Verification items for this drawing (mm, ordinates from the low corner). A direction names the side the tool comes from. Coordinates: 2 decimals unless noted, no trailing zeros. Order: outer loops, then holes, each group sorted by start corner. A loop starts at its lowest first (then second) coordinate and runs counter-clockwise, first axis right, second up. Notation, with made-up numbers: (50, -32.5) -> (91, -32.5) arc R32 ccw to (91, -6.5) -> close; hole circle Ø8 at (49, 88). An arc over 180 degrees is marked (long way). Put each result on its own line as item: value. Start each with the question number.
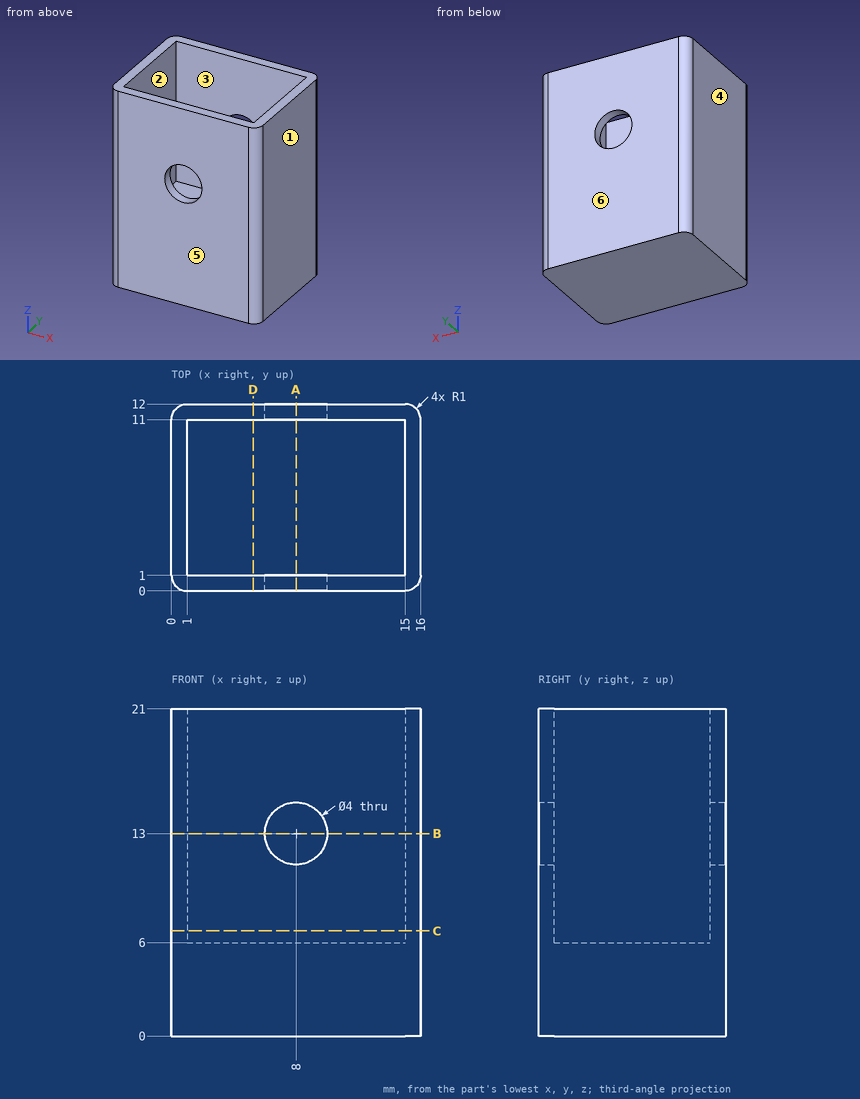
1) Mould release check, pull along Y, two halves, no side actions. Record for the marked faces 3, 4, 5 and 6: +Y half, -Y half, draft (parallel to the pull), parting line (faces both ways), or undercut.
2) Gauge pin test, flat ends, axial feed: pin 1 (4 mm diameter, centred on x = 4, y = 5.5, fed in from +Z); pin 2 (6.5 mm diameter, centred on x = 8, z = 13, fed in from -Y); pin 3 (3.5 mm diameter, centred on x = 8, z = 13, fed in from -Y) (3 decimals). Record the tip position at first contact, or that the pin passes through.
3) Sectioned sample at D-D (x = 5.25). Record the boundary of the cut face in (y, z), plus the area to 3 significant figures.
4) Access from +Z, -Z, +X, -X, +Y, -Y to the whole of each face (thin tool, end or side, straight path). Record for the marked faces 1 and 2.
5) Sectioned sample at A-A (x = 8). Record the boundary of the cut face in (y, z).
6) Sectioned sample at B-B (z = 13). Record the boundary of the cut face in (x, y).
7) Sectioned sample at C-C (z = 6.75). Record the boundary of the cut face in (x, y).
8) Scan lines: line 1 along X through (y, z) = (6, 19.75); line 2 along Z through (x, y) = (8, 11.7); line 3 along Y through (x, z) = (4.5, 8.5). Record each from-to range of solid material in increasing order. Write a range as [from, to].
Entries:
1. face 3: undercut
1. face 4: draft
1. face 5: -Y half
1. face 6: +Y half
2. pin 1: stops at z = 6
2. pin 2: stops at y = 0
2. pin 3: passes through
3. outline: (0, 0) -> (12, 0) -> (12, 21) -> (11, 21) -> (11, 6) -> (1, 6) -> (1, 21) -> (0, 21) -> close
3. area: 102 mm2
4. face 1: +Z, -Z, +X, +Y, -Y
4. face 2: +Z
5. outline: (0, 0) -> (12, 0) -> (12, 11) -> (11, 11) -> (11, 6) -> (1, 6) -> (1, 11) -> (0, 11) -> close; (0, 15) -> (1, 15) -> (1, 21) -> (0, 21) -> close; (11, 15) -> (12, 15) -> (12, 21) -> (11, 21) -> close
6. outline: (0, 1) arc R1 ccw to (1, 0) -> (6, 0) -> (6, 1) -> (1, 1) -> (1, 11) -> (6, 11) -> (6, 12) -> (1, 12) arc R1 ccw to (0, 11) -> close; (10, 0) -> (15, 0) arc R1 ccw to (16, 1) -> (16, 11) arc R1 ccw to (15, 12) -> (10, 12) -> (10, 11) -> (15, 11) -> (15, 1) -> (10, 1) -> close
7. outline: (0, 1) arc R1 ccw to (1, 0) -> (15, 0) arc R1 ccw to (16, 1) -> (16, 11) arc R1 ccw to (15, 12) -> (1, 12) arc R1 ccw to (0, 11) -> close; hole (1, 1) -> (15, 1) -> (15, 11) -> (1, 11) -> close
8. line 1: x = [0, 1], [15, 16]
8. line 2: z = [0, 11], [15, 21]
8. line 3: y = [0, 1], [11, 12]
